Geometry: final body of the model. Coordinates: model frame, mm. A direction names the side the tool comes from. Give positions to 0.01 mm unless a question says otherwise; leave off trailing zeros. Loops run counter-clockwise (first coordinate to the right, second up) from the corner with the lowest first, then second, coordinate; pieces in that order, holes last. Notation, with made-up numbers: (-6, 88.5) -> (-2, 88.5) arc R18 cw to (-2, 112.5) -> close; hole circle Ø7 at (7, -23). An arc over 180 degrees is marked (long way). One line per question, with ' | ' between items. Start each with the question number.
Item 1: Section B-B on x = 49.53. Return loops of the section in (y, z), then the cut area to 3 significant figures.
Item 2: Mould query, pull axis Z, two halves, no side actions, for faces 3 (the cylindrical face through (-6.158, 0.053, 1.55)), 4 (the cylindrical face through (-0.69, -0.05, 3.1)), 5 (the flat face through (32, 0, 8.89)). Classes: released by +Z, released by -Z, zero draft, split by the parting line, or undercut.
Item 3: Section A-A on z = 0. Return loops of the section in (x, y) (3 decimals).
Item 4: Material intervals for line 1 along X through (y, z) = (-2, 0) (3 decimals); line 2 along Z through (x, y) = (0, -2.25) (3 decimals); line 3 along Z through (x, y) = (4, -1), sorted ascending. Write a range as [from, to].
Item 5: Pin query (flat end, axial travel): P1, Ø3.5, axis at x = 48.5, y = -1, coming from the +Z side; P2, Ø2.5, axis at x = 49.53, y = 0, coming from the +Z side. Return the tip coordinate at first contact, or that it passes through.
Item 6: Section C-C on y = -3. Return loops of the section in (x, z) (3 decimals).
Item 7: Section D-D on z = -4. Return loops of the section in (x, y).
Item 8: Set-up query: faces 1 (the flat face through (26, -3.81, 1)), 2 (the flat face through (49, 0, 3.81)). Return all of +Z, -Z, +X, -X, +Y, -Y with unobstructed straight access to the full face (end or side cutting, diameter ignored); none if empty.
from build123d import *

# Parameters (mm, degrees)
SKETCH1_R           = 3.175
BOSS_EXTRUDE1_DEPTH = 3.81
FILLET1_R           = 2.54
SKETCH2_R           = 2.286
SKETCH2_R_2         = 1.89865
CUT_EXTRUDE1_DEPTH  = 5.08


with BuildPart() as part:
    # Sketch1 → Boss-Extrude1 (new body, symmetric)
    with BuildSketch(Plane(origin=(0, 0, 0), x_dir=(1, 0, 0), z_dir=(0, 1, 0))):
        with BuildLine():
            Line((0, 6.35), (12.36646, 6.35))
            Line((12.36646, 6.35), (57.15, 6.35))
            Line((57.15, 6.35), (57.15, -8.89))
            Line((57.15, -8.89), (6.35, -8.89))
            Line((6.35, -8.89), (6.35, 0))
            ThreePointArc((6.35, 0), (-4.490128, -4.490128), (0, 6.35))
        make_face()
        Circle(SKETCH1_R, mode=Mode.SUBTRACT)
    extrude(amount=BOSS_EXTRUDE1_DEPTH, both=True)

    # Fillet1
    fillet1_edges = [part.edges().sort_by_distance(p)[0] for p in [
        (6.35, 0, 0),
    ]]
    fillet(fillet1_edges, radius=FILLET1_R)

    # Sketch2 → Cut-Extrude1 (cut)
    with BuildSketch(Plane.XY.offset(8.89)):
        with Locations((13.97, 0)):
            Circle(SKETCH2_R)
        with Locations((49.53, 0)):
            Circle(SKETCH2_R)
        with Locations((13.97, 0)):
            Circle(SKETCH2_R_2)
        with Locations((49.53, 0)):
            Circle(SKETCH2_R_2)
    extrude(amount=-CUT_EXTRUDE1_DEPTH, mode=Mode.SUBTRACT)


solid = part.part
Result sheet:
1) outline: (-3.81, -6.35) -> (3.81, -6.35) -> (3.81, 8.89) -> (2.29, 8.89) -> (2.29, 3.81) -> (-2.29, 3.81) -> (-2.29, 8.89) -> (-3.81, 8.89) -> close | area: 92.9 mm²
2) face 3: split by the parting line | face 4: undercut | face 5: released by +Z
3) outline: (-6.35, -3.81) -> (-3.175, -3.81) -> (-3.175, 3.81) -> (-6.35, 3.81) -> close; (3.175, -3.81) -> (57.15, -3.81) -> (57.15, 3.81) -> (3.175, 3.81) -> close
4) line 1: x = [-6.35, -3.175], [3.175, 57.15] | line 2: z = [-6.35, -3.175], [3.175, 6.35] | line 3: z = [-6.35, 5.5]
5) P1: stops at z = 8.89 | P2: stops at z = 3.81
6) outline: (0, -6.35) -> (57.15, -6.35) -> (57.15, 8.89) -> (6.35, 8.89) -> (6.35, 8.032) arc R2.54 cw to (2.721, 5.737) arc R6.35 ccw (long way) to start; hole circle Ø6.35 at (0, 0)
7) outline: (-4.93, -3.81) -> (57.15, -3.81) -> (57.15, 3.81) -> (-4.93, 3.81) -> close
8) face 1: +Z, -Z, +X, -X, -Y | face 2: +Z
